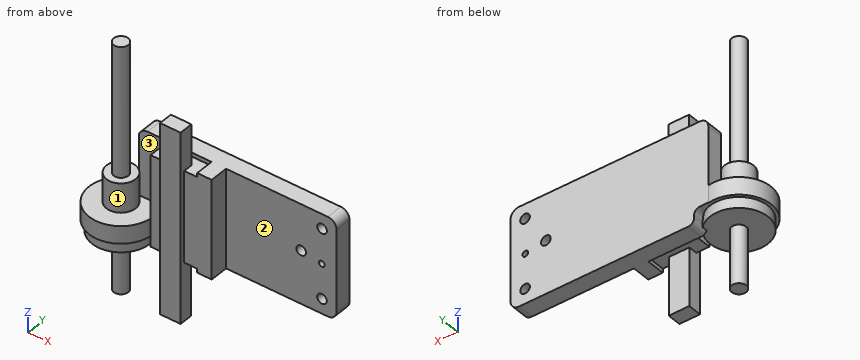
from build123d import *

# Parameters (mm, degrees)
BOSS_EXTRUDE1_DEPTH             = 7.2517
FILLET1_R                       = 2.54
SKETCH3_W                       = 6.3246
SKETCH3_H                       = 43.2054
BOSS_EXTRUDE2_DEPTH             = 8.0264
SKETCH4_W                       = 20.32
SKETCH4_H                       = 39.7256
BOSS_EXTRUDE3_DEPTH             = 8.0264
SKETCH5_W                       = 8.9535
SKETCH5_H                       = 39.7256
BOSS_EXTRUDE4_DEPTH             = 2.032
BOSS_EXTRUDE5_DEPTH             = 7.62
SKETCH7_R                       = 12.6365
BOSS_EXTRUDE6_DEPTH             = 4.7625
SKETCH8_R                       = 6.35
BOSS_EXTRUDE7_DEPTH             = 12.7
SKETCH10_R                      = 3.175
BOSS_EXTRUDE8_DEPTH             = 56.642
BOSS_EXTRUDE9_START             = 25.4
SKETCH12_R                      = 3.175
BOSS_EXTRUDE9_DEPTH             = 25.4
SKETCH15_W                      = 8.9535
SKETCH15_H                      = 6.039178017
BOSS_EXTRUDE12_DEPTH            = 17.78
SKETCH14_W                      = 8.9535
SKETCH14_H                      = 5.969
BOSS_EXTRUDE13_DEPTH            = 25.4
TAP_DRILL_FOR_M5X0_8_TAP1_D     = 4.2
TAP_DRILL_FOR_M5X0_8_TAP1_DEPTH = 25.4
TAP_DRILL_FOR_M5X0_8_TAP1_TIP   = 1.2618073
TAP_DRILL_FOR_M3X0_5_TAP1_D     = 2.5
TAP_DRILL_FOR_M3X0_5_TAP1_DEPTH = 25.4
TAP_DRILL_FOR_M3X0_5_TAP1_TIP   = 0.751075774
TAP_DRILL_FOR_M5X0_8_TAP2_D     = 4.2
TAP_DRILL_FOR_M5X0_8_TAP2_DEPTH = 25.4
TAP_DRILL_FOR_M5X0_8_TAP2_TIP   = 1.2618073


with BuildPart() as part:
    # Sketch1 → Boss-Extrude1 (new body)
    with BuildSketch(Plane(origin=(0, 0, 0), x_dir=(1, 0, 0), z_dir=(0, 1, 0))):
        with BuildLine():
            Line((39.37, 21.6027), (-36.9824, 21.6027))
            Line((-36.9824, 21.6027), (-36.9824, 15.2527))
            Line((-36.9824, 15.2527), (-36.9824, -21.6027))
            Line((-36.9824, -21.6027), (39.37, -21.6027))
            ThreePointArc((39.37, -21.6027), (42.064076836, -20.486776836), (43.18, -17.7927))
            Line((43.18, -17.7927), (43.18, 17.7927))
            ThreePointArc((43.18, 17.7927), (42.064076836, 20.486776836), (39.37, 21.6027))
        make_face()
        with BuildLine():
            Line((-36.9824, -21.6027), (-36.9824, 15.2527))
            Line((-36.9824, 15.2527), (-43.18, 15.2527))
            Line((-43.18, 15.2527), (-43.18, -17.7927))
            ThreePointArc((-43.18, -17.7927), (-42.064076836, -20.486776836), (-39.37, -21.6027))
            Line((-39.37, -21.6027), (-36.9824, -21.6027))
        make_face()
    extrude(amount=BOSS_EXTRUDE1_DEPTH)

    # Fillet1
    fillet1_edges = [part.edges().sort_by_distance(p)[0] for p in [
        (-36.9824, 3.62585, -15.2527),
        (-36.9824, 3.62585, -21.6027),
    ]]
    fillet(fillet1_edges, radius=FILLET1_R)

    # Sketch3 → Boss-Extrude2 (add)
    with BuildSketch(Plane.XZ):
        with Locations((-8.2423, 0)):
            Rectangle(SKETCH3_W, SKETCH3_H)
    extrude(amount=BOSS_EXTRUDE2_DEPTH)

    # Sketch4 → Boss-Extrude3 (add)
    with BuildSketch(Plane.XZ):
        with Locations((-21.5646, 0)):
            Rectangle(SKETCH4_W, SKETCH4_H)
    extrude(amount=BOSS_EXTRUDE3_DEPTH)

    # Sketch5 → Boss-Extrude4 (add)
    with BuildSketch(Plane.XZ.offset(8.0264)):
        with Locations((-21.5646, 0)):
            Rectangle(SKETCH5_W, SKETCH5_H)
    extrude(amount=BOSS_EXTRUDE4_DEPTH)

    # Sketch6 → Boss-Extrude5 (add)
    with BuildSketch(Plane(origin=(0, 0, -15.2527), x_dir=(-1, 0, 0), z_dir=(0, 0, -1))):
        with BuildLine():
            Line((31.7246, 0), (31.7246, -6.7183))
            ThreePointArc((31.7246, -6.7183), (59.227378961, -10.185978415), (33.44611662, 0))
            Line((33.44611662, 0), (31.7246, 0))
        make_face()
    extrude(amount=-BOSS_EXTRUDE5_DEPTH)

    # Sketch7 → Boss-Extrude6 (add)
    with BuildSketch(Plane(origin=(0, 0, -15.2527), x_dir=(-1, 0, 0), z_dir=(0, 0, -1))):
        with Locations((45.6946, -6.7183)):
            Circle(SKETCH7_R)
    extrude(amount=BOSS_EXTRUDE6_DEPTH)

    # Sketch8 → Boss-Extrude7 (add)
    with BuildSketch(Plane.XY.offset(-7.6327)):
        with Locations(Location((-45.6946, -6.7183, 0), (0, 0, 180))):
            Circle(SKETCH8_R)
    extrude(amount=BOSS_EXTRUDE7_DEPTH)

    # Sketch10 → Boss-Extrude8 (add)
    with BuildSketch(Plane.XY.offset(5.0673)):
        with Locations((-45.6946, -6.7183)):
            Circle(SKETCH10_R)
    extrude(amount=BOSS_EXTRUDE8_DEPTH)

    # Sketch12 → Boss-Extrude9 (add)
    with BuildSketch(Plane(origin=(0, 0, -20.0152), x_dir=(-1, 0, 0), z_dir=(0, 0, -1)).offset(BOSS_EXTRUDE9_START)):
        with Locations(Location((45.6946, -6.7183, 0), (0, 0, 180))):
            Circle(SKETCH12_R)
    extrude(amount=-BOSS_EXTRUDE9_DEPTH)

    # Sketch15 → Boss-Extrude12 (add)
    with BuildSketch(Plane.XY.offset(19.8628)):
        with Locations((-21.5646, -7.038810992)):
            Rectangle(SKETCH15_W, SKETCH15_H)
    extrude(amount=BOSS_EXTRUDE12_DEPTH)

    # Sketch14 → Boss-Extrude13 (add)
    with BuildSketch(Plane(origin=(0, 0, -19.8628), x_dir=(-1, 0, 0), z_dir=(0, 0, -1))):
        with Locations((21.5646, -7.0739)):
            Rectangle(SKETCH14_W, SKETCH14_H)
    extrude(amount=BOSS_EXTRUDE13_DEPTH)

    # Tap Drill for M5x0.8 Tap1
    with Locations(Plane(origin=(0, 7.2517, 0), x_dir=(1, 0, 0), z_dir=(0, 1, 0))):
        with Locations((36.8046, 15.1511), (36.83, -15.2527)):
            Hole(TAP_DRILL_FOR_M5X0_8_TAP1_D / 2, depth=TAP_DRILL_FOR_M5X0_8_TAP1_DEPTH)
            with Locations((0, 0, -(TAP_DRILL_FOR_M5X0_8_TAP1_DEPTH + TAP_DRILL_FOR_M5X0_8_TAP1_TIP / 2))):  # 118° drill point
                Cone(0, TAP_DRILL_FOR_M5X0_8_TAP1_D / 2, TAP_DRILL_FOR_M5X0_8_TAP1_TIP, mode=Mode.SUBTRACT)

    # Tap Drill for M3x0.5 Tap1
    with Locations(Plane(origin=(0, 7.2517, 0), x_dir=(1, 0, 0), z_dir=(0, 1, 0))):
        with Locations((36.703, 0)):
            Hole(TAP_DRILL_FOR_M3X0_5_TAP1_D / 2, depth=TAP_DRILL_FOR_M3X0_5_TAP1_DEPTH)
            with Locations((0, 0, -(TAP_DRILL_FOR_M3X0_5_TAP1_DEPTH + TAP_DRILL_FOR_M3X0_5_TAP1_TIP / 2))):  # 118° drill point
                Cone(0, TAP_DRILL_FOR_M3X0_5_TAP1_D / 2, TAP_DRILL_FOR_M3X0_5_TAP1_TIP, mode=Mode.SUBTRACT)

    # Tap Drill for M5x0.8 Tap2
    with Locations(Plane(origin=(0, 7.2517, 0), x_dir=(1, 0, 0), z_dir=(0, 1, 0))):
        with Locations((27.7241, -1.5367)):
            Hole(TAP_DRILL_FOR_M5X0_8_TAP2_D / 2, depth=TAP_DRILL_FOR_M5X0_8_TAP2_DEPTH)
            with Locations((0, 0, -(TAP_DRILL_FOR_M5X0_8_TAP2_DEPTH + TAP_DRILL_FOR_M5X0_8_TAP2_TIP / 2))):  # 118° drill point
                Cone(0, TAP_DRILL_FOR_M5X0_8_TAP2_D / 2, TAP_DRILL_FOR_M5X0_8_TAP2_TIP, mode=Mode.SUBTRACT)


solid = part.part
The model under review builds one solid part; all positions refer to its coordinate system, in mm. Face numbers are marked on the shaded views. A direction names the side the tool comes from. Coordinates: 2 decimals unless noted, no trailing zeros. Order: outer loops, then holes, each group sorted by start corner. A loop starts at its lowest first (then second) coordinate and runs counter-clockwise, first axis right, second up. Notation, with made-up numbers: (21, -29.75) -> (32, -29.75) arc R23 cw to (32, 3.25) -> close; hole circle Ø8 at (-33.75, 88.5). An arc over 180 degrees is marked (long way). Answer in a Markdown table with one row per item.
(1) Consider section C-C (x = 27). Write out the cut boundary in (y, z).
Answers:
| item | result |
|---|---|
| outline | (0, -21.6) -> (7.25, -21.6) -> (7.25, -0.43) -> (0, -0.43) -> close; (0, 3.51) -> (7.25, 3.51) -> (7.25, 21.6) -> (0, 21.6) -> close |
(2) Machinability: for the marked faces 1, 2 and 3, which of the approach directions +Z, -Z, +X, -X, +Y, -Y give a long, thin tool a straight path to every point of the face, cutting with its end or side? Answer none if there is none.
Answers:
| item | result |
|---|---|
| face 1 | +Z |
| face 2 | +Z, -Z, +X, -Y |
| face 3 | +Z, -X |
(3) Consider section B-B (y = -14.5). Write out the cut boundary in (x, z).
Answers:
| item | result |
|---|---|
| outline | (-57.3, -15.25) -> (-55.65, -15.25) -> (-55.65, -20.02) -> (-35.74, -20.02) -> (-35.74, -15.25) -> (-34.09, -15.25) -> (-34.09, -7.63) -> (-57.3, -7.63) -> close |
(4) Consider section A-A (x = -29.5). Write out the cut boundary in (y, z), plus the area to 3 significant figures.
Answers:
| item | result |
|---|---|
| outline | (-8.03, -19.86) -> (0, -19.86) -> (0, -21.6) -> (7.25, -21.6) -> (7.25, 21.6) -> (0, 21.6) -> (0, 19.86) -> (-8.03, 19.86) -> close |
| area | 632 mm² |
(5) Wall thickness on line 1 along Z through (x, y) = (36.83, 2.5); line 2 along X through (y, z) = (-6.75, 11); line 3 along Y through (x, z) = (20, -11.5): over which ranges is each line inside the solid? List them lowest first.
Answers:
| item | result |
|---|---|
| line 1 | -21.6 to -17.25, -13.05 to -1.24, 1.24 to 13.15, 17.35 to 21.6 |
| line 2 | -48.87 to -42.52, -31.72 to -5.08 |
| line 3 | 0 to 7.25 |
(6) Insertion check: pin 1 (1 mm diameter, centred on y = 5.5, z = -18.5, fed in from -X); pin 2 (5 mm diameter, centred on x = -21.5, y = -7, fed in from -Z); pin 3 (5 mm diameter, centred on x = -3.5, y = -8.5, fed in from +Z); pin 4 (3 mm diameter, centred on x = -31.5, y = -13.5, fed in from +Z). Each pin has a flat end and moves straight along its axis. Give the tip position at first contact, or say it passes through.
Answers:
| item | result |
|---|---|
| pin 1 | x = -50.42 |
| pin 2 | z = -45.26 |
| pin 3 | z = 21.6 |
| pin 4 | through |
